Autodesk Inventor part; units mm, degrees
ref_plane "Pracovní rovina1" through (0, 14, 0) normal (0, 1, 0) x (-1, 0, 0)
ref_plane "YZ Plane" through (0, 0, 0) normal (1, 0, 0) x (0, 1, 0)
ref_plane "XZ Plane" through (0, 0, 0) normal (0, 1, 0) x (-1, 0, 0)
sketch "Náčrt1" plane through (0, 0, 0) normal (0, 0, 1) x (1, 0, 0)
  line L0 (11, 8.6603) -> (11, -8.6603)
  line L1 (-11, -8.6603) -> (-11, 8.6603)
  arc A0 (-11, -8.6603) -> (11, -8.6603) centre (0, 0) ccw
  line L2 (-4, 13.4164) -> (-4, 10)
  line L3 (-4, 10) -> (-6, 10)
  line L4 (-6, 6) -> (6, 6)
  line L5 (6, 10) -> (4, 10)
  line L6 (4, 10) -> (4, 13.4164)
  line L7 (-6, 10) -> (-6, 6)
  line L8 (6, 10) -> (6, 6)
  arc A1 (11, 8.6603) -> (4, 13.4164) centre (0, 0) ccw
  arc A2 (-4, 13.4164) -> (-11, 8.6603) centre (0, 0) ccw
  dimension "d26" = 22
  dimension "attachmentRadius" = 14
  dimension "d28" = 14
  dimension "d29" = 14
extrude "Vysunutí1" add sketch "Náčrt1" along normal blind 20
ref_plane "Pracovní rovina1" through (0, 14, 0) normal (0, 1, 0) x (-1, 0, 0)
sketch "Náčrt2" plane through (0, 14, 0) normal (0, 1, 0) x (-1, 0, 0)
  line L0 (11, 0) -> (11, 20)
  line L1 (4, 0) -> (4, 20)
  line L2 (11, 16) -> (4, 16)
  line L3 (4, 16) -> (4, 12)
  line L4 (4, 12) -> (11, 12)
  line L5 (11, 12) -> (11, 16)
  line L6 (-4, 0) -> (-4, 20)
  line L7 (-11, 0) -> (-11, 20)
  line L8 (-4, 16) -> (-11, 16)
  line L9 (-11, 16) -> (-11, 12)
  line L10 (-11, 12) -> (-4, 12)
  line L11 (-4, 12) -> (-4, 16)
  point P0 (0, 0)
extrude "Vysunutí2" cut sketch "Náčrt2" against normal up to next
sketch "Náčrt6" plane through (0, 0, 20) normal (0, 0, 1) x (1, 0, 0)
  circle A0 centre (7.5, 0) radius 1.5
  circle A1 centre (-7.5, 0) radius 1.5
  line L0 (11, -8.6603) -> (11, 8.6603)
  line L1 (-11, 8.6603) -> (-11, -8.6603)
  arc A2 (11, 8.6603) -> (4, 13.4164) centre (0, 0) ccw
  dimension "d15" = 3.5
  dimension "attachmentHoleOffset" = 3.5
  dimension "d17" = 3
  dimension "attachmentHoleDia" = 3
extrude "Vysunutí6" cut sketch "Náčrt6" against normal up to surface (20 mm away)
sketch "Náčrt8" plane through (0, 0, 0) normal (0, 0, -1) x (-1, 0, 0)
  circle A0 centre (-7.5, 0) radius 1.5
  circle A1 centre (7.5, 0) radius 1.5
  line L0 (-11, 8.6603) -> (-11, -8.6603)
  arc A2 (-11, -8.6603) -> (11, -8.6603) centre (0, 0) ccw
  line L1 (11, -8.6603) -> (11, 8.6603)
  arc A3 (11, 8.6603) -> (4, 13.4164) centre (0, 0) ccw
  line L2 (4, 13.4164) -> (4, 10)
  line L3 (4, 10) -> (6, 10)
  line L4 (6, 10) -> (6, 6)
  line L5 (6, 6) -> (-6, 6)
  line L6 (-6, 6) -> (-6, 10)
  line L7 (-6, 10) -> (-4, 10)
  line L8 (-4, 10) -> (-4, 13.4164)
  arc A4 (-4, 13.4164) -> (-11, 8.6603) centre (0, 0) ccw
extrude "Vysunutí8" cut sketch "Náčrt8" against normal blind 4
sketch "Náčrt9" plane through (0, 0, 20) normal (0, 0, 1) x (1, 0, 0)
  arc A0 (-4, 13.4164) -> (-11, 8.6603) centre (0, 0) ccw
  circle A1 centre (0, 0) radius 3
extrude "Vysunutí9" cut sketch "Náčrt9" against normal up to next
sketch "Náčrt10" plane through (0, 0, 20) normal (0, 0, 1) x (1, 0, 0)
  circle A0 centre (0, 0) radius 3
  arc A1 (-11, -8.6603) -> (11, -8.6603) centre (0, 0) ccw
  circle A2 centre (0, 0) radius 4
  dimension "d23" = 8
extrude "Vysunutí10" cut sketch "Náčrt10" against normal blind 3
sketch "Náčrt11" plane through (0, 0, 20) normal (0, 0, 1) x (1, 0, 0)
  circle A0 centre (7.5, 0) radius 1.5
  circle A1 centre (-7.5, 0) radius 1.5
  circle A2 centre (-7.5, 0) radius 1.5
  circle A3 centre (-7.5, 0) radius 2.75
  circle A4 centre (7.5, 0) radius 1.5
  circle A5 centre (7.5, 0) radius 2.75
  dimension "d30" = 5.5
  dimension "d31" = 5.5
extrude "Vysunutí11" cut sketch "Náčrt11" against normal blind 1.5
sketch "Náčrt12" plane through (0, 0, 4) normal (0, 0, -1) x (-1, 0, 0)
  line L0 (7.5, 3.1754) -> (10.25, 1.5877)
  line L1 (10.25, 1.5877) -> (10.25, -1.5877)
  line L2 (10.25, -1.5877) -> (7.5, -3.1754)
  line L3 (7.5, -3.1754) -> (4.75, -1.5877)
  line L4 (4.75, -1.5877) -> (4.75, 1.5877)
  line L5 (4.75, 1.5877) -> (7.5, 3.1754)
  line L6 (-11, -8.6603) -> (-11, 8.6603)
  circle A0 centre (-7.5, 0) radius 1.5
  line L7 (-7.5, 3.1754) -> (-4.75, 1.5877)
  line L8 (-4.75, 1.5877) -> (-4.75, -1.5877)
  line L9 (-4.75, -1.5877) -> (-7.5, -3.1754)
  line L10 (-7.5, -3.1754) -> (-10.25, -1.5877)
  line L11 (-10.25, -1.5877) -> (-10.25, 1.5877)
  line L12 (-10.25, 1.5877) -> (-7.5, 3.1754)
  point P0 (7.5, 0)
  point P1 (7.5, 0)
  dimension "d38" = 5.5
extrude "Vysunutí13" cut sketch "Náčrt12" against normal blind 2.4
equation "\"d28\" = attachmentRadius"
equation "\"d29\" = attachmentRadius"
equation "\"d15\" = attachmentHoleOffset"
equation "\"d17\" = attachmentHoleDia"
properties part number "attachment"
Can you work these out from the model? Positions are in its coordinate system, mm. A direction names the side the tool comes from. Give positions to 0.01 mm unless a question says otherwise; leave off trailing zeros. Loops run counter-clockwise (first coordinate to the right, second up) from the corner with the lowest first, then second, coordinate; pieces in that order, holes last. Notation, with made-up numbers: M 49,72.25 L 68,72.25 A28 cw 68,106.25 Z; hole C 37,5.25 d1. An arc over 180 degrees is marked long. One line per item, written item: value. Start each with the question number.
1) If we section it at A-A, the plane x = 0: Write out the boundary of the cut face in (y, z).
2) I'm going to push flat-ended pins straight in: pin 1 (5 mm diameter, centred on x = 7.5, y = 0, fed in from -Z); pin 2 (1 mm diameter, centred on y = 11.5, z = 18.5, fed in from -X); pin 3 (0.6 mm diameter, centred on x = 5.5, z = 18.5, fed in from -Y). Where does each tip first touch, or does it pass through?
3) Thinking about a two-plate mould opening in X: for faces 5 (the face through (-6, 8, 18)), 6 (the face through (-7.918, 11.546, 17.972)), 7 (the face through (0.15, -3.15, 4)), which applies, +X half, -X half, draft (parallel to the pull), parting line (faces both ways), or undercut?
4) If we section it at B-B, the plane y = 5: Write out the boundary of the cut face in (x, z).
5) On a 3-axis mill with a long thin cutter (end or side, diameter ignored), from which of +Z, -Z, +X, -X, +Y, -Y can I reach the whole of each face in a straight line? I mean faces 1 (the face through (-6, -1, 18.5)), 2 (the face through (8.894, 2.37, 5.183)), 3 (the face through (-4, 12, 8)), 4 (the face through (-5, 10, 18)). Say none if no direction works.
6) If we section it at D-D, the plane x = -6.75: Write out the boundary of the cut face in (y, z).
7) If I drill on line 1 (Z direction, x = -4.75, y = 11.5); line 2 (Z direction, x = 9, y = 1.5); line 3 (X direction, y = 6.75, z = 7.5), over which ranges is the centre line in solid material (lowest first)? Write a range as [from, to].
8) If we section it at C-C, the plane z = 15.5: Write out the boundary of the cut face in (x, y), and give its area (3 significant figures).
Completed:
1. outline: M -14,4 L -3,4 L -3,17 L -4,17 L -4,20 L -14,20 Z; M 3,4 L 6,4 L 6,20 L 4,20 L 4,17 L 3,17 Z
2. pin 1: stops at z = 6.4
2. pin 2: stops at x = -8.66
2. pin 3: stops at y = -13
3. face 5: undercut
3. face 6: -X half
3. face 7: draft
4. outline: M -11,4 L 11,4 L 11,12 L 4,12 L 4,16 L 11,16 L 11,20 L -11,20 L -11,16 L -4,16 L -4,12 L -11,12 Z
5. face 1: +Z
5. face 2: -Z
5. face 3: +Z, -Z, +Y
5. face 4: +Z, -Z
6. outline: M -12.27,4 L -2.74,4 L -2.74,6.4 L -1.3,6.4 L -1.3,12 L -12.27,12 Z; M -12.27,16 L -1.3,16 L -1.3,18.5 L -2.65,18.5 L -2.65,20 L -12.27,20 Z; M 1.3,6.4 L 2.74,6.4 L 2.74,4 L 12.27,4 L 12.27,12 L 1.3,12 Z; M 1.3,16 L 12.27,16 L 12.27,20 L 2.65,20 L 2.65,18.5 L 1.3,18.5 Z
7. line 1: z = [4, 12], [16, 20]
7. line 2: z = [6.4, 12], [16, 18.5]
7. line 3: x = [-11, -6], [6, 11]
8. outline: M -4,-13.42 A14 ccw 4,-13.42 L 4,6 L -4,6 Z; hole C 0,0 d6
8. area: 130 mm^2
